Build history of the part. All positions in model axes, mm. A direction names the side the tool comes from. Give positions to 0.01 mm unless a question says otherwise; leave off trailing zeros. Order: outer loops, then holes, each group sorted by start corner. A loop starts at its lowest first (then second) coordinate and runs counter-clockwise, first axis right, second up. Notation, with made-up numbers: M 48,57 L 89,57 A35 cw 89,95 Z; hole C 79,-32 d9. An arc over 180 degrees is marked long. One line per item, written item: value.
from build123d import *

# Parameters (mm, degrees)
SKETCH1_R           = 12.7
BOSS_EXTRUDE1_DEPTH = 19.05
SKETCH2_R           = 15.875
BOSS_EXTRUDE2_DEPTH = 3.175
SKETCH3_R           = 15.875
BOSS_EXTRUDE3_DEPTH = 3.175
SKETCH4_R           = 6.35
CUT_EXTRUDE1_DEPTH  = 26.4
FILLET1_R           = 1.27


with BuildPart() as part:
    # Sketch1 → Boss-Extrude1 (new body)
    with BuildSketch(Plane(origin=(0, 0, 0), x_dir=(0, 0, -1), z_dir=(1, 0, 0))):
        Circle(SKETCH1_R)
    extrude(amount=BOSS_EXTRUDE1_DEPTH)

    # Sketch2 → Boss-Extrude2 (add)
    with BuildSketch(Plane.ZY):
        Circle(SKETCH2_R)
    extrude(amount=BOSS_EXTRUDE2_DEPTH)

    # Sketch3 → Boss-Extrude3 (add)
    with BuildSketch(Plane(origin=(19.05, 0, 0), x_dir=(0, 0, -1), z_dir=(1, 0, 0))):
        Circle(SKETCH3_R)
    extrude(amount=BOSS_EXTRUDE3_DEPTH)

    # Sketch4 → Cut-Extrude1 (cut, through all)
    with BuildSketch(Plane.ZY.offset(3.175)):
        Circle(SKETCH4_R)
    extrude(amount=-CUT_EXTRUDE1_DEPTH, mode=Mode.SUBTRACT)

    # Fillet1
    fillet1_edges = [part.edges().sort_by_distance(p)[0] for p in [
        (0, 0, -15.875),
        (19.05, 0, 15.875),
    ]]
    fillet(fillet1_edges, radius=FILLET1_R)


solid = part.part
1) Pin check, flat tips, straight feed: pin 1 (6 mm diameter, centred on x = 15, y = -6.5, fed in from -Z); pin 2 (3 mm diameter, centred on x = 8, z = 0, fed in from -Y); pin 3 (3 mm diameter, centred on x = 18.5, y = -9.5, fed in from +Z). Stop position of each tip, or through.
Check values:
pin 1: z = -12.21
pin 2: y = -12.7
pin 3: z = 13.16
2) Saw through at C-C, the plane x = 3. Write the cut outline in (y, z), then the cut area to 3 significant figures.
Check values:
outline: C 0,0 d25.4; hole C 0,0 d12.7
area: 380 mm^2
3) Tool access for faces 4 (the face through (9.35, -6.2, -1.38)), 5 (the face through (9.39, -12.4, 2.75)): list every direction of +Z, -Z, +X, -X, +Y, -Y with a clear straight run to the whole face (end or side of a thin tool).
Check values:
face 4: +X, -X
face 5: none
4) Drill centre lines: probe 1 along Y at (x, z) = (6.75, 0); probe 2 along X at (y, z) = (-14, 4) (3 decimals); probe 3 along Z at (x, y) = (15, 2.5). Where is each one in solid material? Low to high. Write a range as from..to.
Check values:
probe 1: -12.7..-6.35, 6.35..12.7
probe 2: -3.175..0, 19.05..22.225
probe 3: -12.45..-5.84, 5.84..12.45
5) Saw through at D-D, the plane x = 19.75. Write the cut outline in (y, z), then the cut area to 3 significant figures.
Check values:
outline: C 0,0 d31.48; hole C 0,0 d12.7
area: 652 mm^2
6) Mould opens along X. For faces 1 (the face through (-2.209, -15.497, -3.441)), 2 (the face through (-3.175, 0, 7)), 3 (the face through (19.05, 7, 11)) say: released by +X, released by -X, zero draft, split by the parting line, or undercut.
Check values:
face 1: zero draft
face 2: released by -X
face 3: undercut
7) Saw through at A-A, the plane z = 0. Write the cut outline in (x, y) (3 decimals).
Check values:
outline: M -3.175,-15.875 L -1.27,-15.875 A1.27 ccw 0,-14.605 L 0,-12.7 L 19.05,-12.7 L 19.05,-14.605 A1.27 ccw 20.32,-15.875 L 22.225,-15.875 L 22.225,-6.35 L -3.175,-6.35 Z; M -3.175,6.35 L 22.225,6.35 L 22.225,15.875 L 20.32,15.875 A1.27 ccw 19.05,14.605 L 19.05,12.7 L 0,12.7 L 0,14.605 A1.27 ccw -1.27,15.875 L -3.175,15.875 Z
